Source: CAD feature listing. Evaluate the final solid. Frame: model axes, mm. Face numbers are marked on the shaded views. A direction names the side the tool comes from. Coordinates: 2 decimals unless noted, no trailing zeros. Order: outer loops, then holes, each group sorted by start corner. A loop starts at its lowest first (then second) coordinate and runs counter-clockwise, first axis right, second up. Notation, with made-up numbers: (75.25, 10.25) - (93.25, 10.25) arc R20 cw to (93.25, 38.25) - close; hole circle Ø4 at (62.25, 55.25). An arc over 180 degrees is marked (long way). One line per question, with ' | ' between items. Start each with the question number.
(1) Access query for the marked faces 1, 2 and 3. Directions: +Z, -Z, +X, -X, +Y, -Y. A direction counts if a zero-diameter tool reaches every point of the face in a straight line with its end or side. Return the directions, or none.
(2) Line query: line 1 along Y through (x, z) = (-0.25, -1.6); line 2 along X through (y, z) = (3, -0.95); line 3 along Y through (x, z) = (-3, -0.5). Output: solid intervals per line, ascending.
(3) Section A-A (z = -0.9). Return the cut outline in (x, y).
(4) Contact query for flat-ended pins moving along their axis: P1, Ø1, axis at y = 5, z = -2, coming from the -X side; P2, Ø1.1, axis at x = 11, z = -2, coming from the -Y side; P3, Ø0.6, axis at x = -7, z = -1.5, coming from the +Y side. Output: stop coordinate, or through.
(5) Section C-C (y = -6). Return the cut outline in (x, z), then the cut area to 3 significant figures.
(6) Section B-B (x = 4.25). Return the cut outline in (y, z).
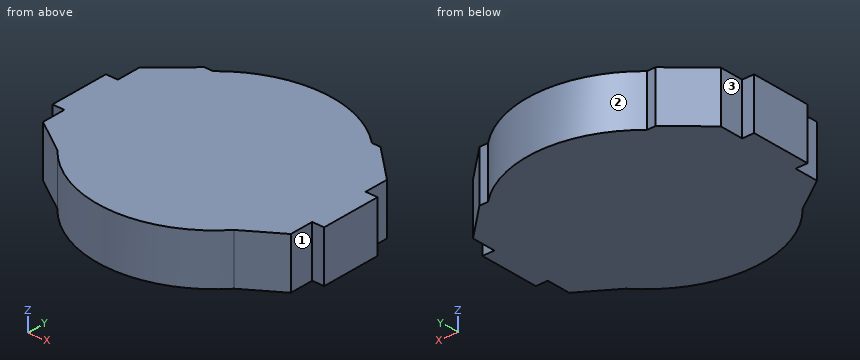
from build123d import *

# Parameters (mm, degrees)
F1_DEPTH = 4.318


with BuildPart() as f1:
    # F0 (on Top) → F1 (new body)
    with BuildSketch(Plane.XY):
        Polygon((-10.541, 2.54), (-11.557, 2.54), (-11.557, -2.54), (-10.541, -2.54), (-10.541, -4.572), (-7.515558, -6.588961), (-5.588, -7.874), (0, -7.874), (5.588, -7.874), (7.515558, -6.588961), (10.541, -4.572), (10.541, -2.54), (11.557, -2.54), (11.557, 2.54), (10.541, 2.54), (10.541, 4.572), (7.493, 7.366), (6.755743, 7.366), (0, 7.366), (-6.755743, 7.366), (-7.493, 7.366), (-10.541, 4.572), align=None)
        with BuildLine():
            ThreePointArc((6.755743, 7.366), (0, 9.9949), (-6.755743, 7.366))
            Line((-6.755743, 7.366), (0, 7.366))
            Line((0, 7.366), (6.755743, 7.366))
        make_face()
        with BuildLine():
            Line((-5.588, -7.874), (-7.515558, -6.588961))
            ThreePointArc((-7.515558, -6.588961), (0, -9.9949), (7.515558, -6.588961))
            Line((7.515558, -6.588961), (5.588, -7.874))
            Line((5.588, -7.874), (0, -7.874))
            Line((0, -7.874), (-5.588, -7.874))
        make_face()
    extrude(amount=-F1_DEPTH)


solid = f1.part
Response values:
1) face 1: +Z, -Z, +X, -Y | face 2: +Z, -Z, +Y | face 3: +Z, -Z, -X, +Y
2) line 1: y = -9.99 to 9.99 | line 2: x = -10.54 to 10.54 | line 3: y = -9.53 to 9.53
3) outline: (-11.56, -2.54) - (-10.54, -2.54) - (-10.54, -4.57) - (-7.52, -6.59) arc R9.99 ccw to (7.52, -6.59) - (10.54, -4.57) - (10.54, -2.54) - (11.56, -2.54) - (11.56, 2.54) - (10.54, 2.54) - (10.54, 4.57) - (7.49, 7.37) - (6.76, 7.37) arc R9.99 ccw to (-6.76, 7.37) - (-7.49, 7.37) - (-10.54, 4.57) - (-10.54, 2.54) - (-11.56, 2.54) - close
4) P1: stops at x = -10.54 | P2: stops at y = -4.63 | P3: stops at y = 7.42
5) outline: (-8.4, -4.32) - (8.4, -4.32) - (8.4, 0) - (-8.4, 0) - close | area: 72.5 mm²
6) outline: (-9.05, -4.32) - (9.05, -4.32) - (9.05, 0) - (-9.05, 0) - close
